Input: part model. Units: mm. Frame: model coordinates. Face numbers are marked on the shaded views. A direction names the side the tool comes from. Round coordinates to 2 decimals unless told otherwise and drop trailing zeros. Loops run counter-clockwise (first coordinate to the right, second up) from the corner with the lowest first, then second, coordinate; pieces in that order, holes last.
(1) Cut plane D-D, the plane z = -2.3. Output: boundary loops of the cut face in (x, y), and give its area (3 significant figures).
(2) Line query: line 1 (Y direction, x = -8, z = 1.85); line 2 (Y direction, x = 6.5, z = 0.9); line 3 (Z direction, x = 4, y = 4.5). Output: solid intervals per line, ascending.
(3) Cut plane A-A, the plane y = 0. Output: boundary loops of the cut face in (x, z), and give its area (3 significant figures).
(4) Access query for the marked faces 4, 5 and 6. Directions: +Z, -Z, +X, -X, +Y, -Y. A direction counts if a zero-diameter tool reaches every point of the face in a straight line with its end or side. Return the directions, or none.
(5) First-contact query: pin 1 Ø6 at (x, y) = (-5.5, 4) entering from +Z; pin 2 Ø4.5 at (x, y) = (-0.5, -1) entering from -Z; pin 3 Ø3 at (x, y) = (0, -7.25) entering from +Z; pin 4 Ø3 at (x, z) = (3.5, 0.5) entering from +Y. Flat tips, straight axial feed; report the tip coordinate or a pass-through.
(6) Draft query along X for the marked faces 1, 2 and 3. Return one class per face: released by +X, released by -X, zero draft, split by the parting line, or undercut.
(7) Cut plane C-C, the plane z = 1.1. Give the number of separate pieces and of enclosed holes in the cut face, and give its area (3 significant figures).
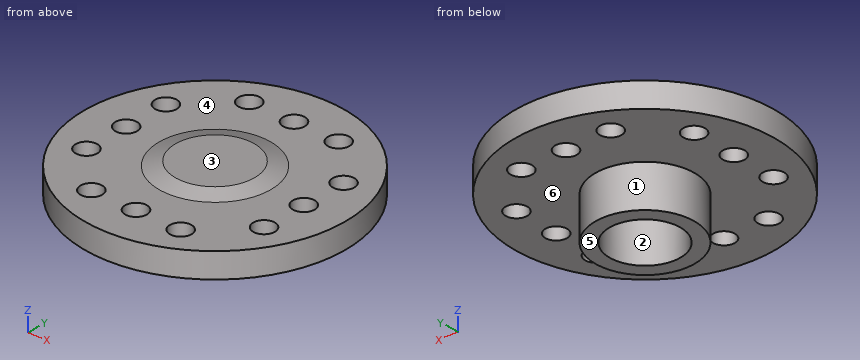
from build123d import *

# Parameters (mm, degrees)
ESQUISSE1_R             = 10.5
ESQUISSE1_R_2           = 0.875
BOSS_EXTRU_1_DEPTH      = 2
ESQUISSE2_R             = 4.5
BOSS_EXTRU_2_DEPTH      = 0.35
BOSS_EXTRU_2_TAPER      = 75
ESQUISSE3_R             = 4
BOSS_EXTRU_3_DEPTH      = 3.4
ESQUISSE4_R             = 2.85
ENL_V_MAT_EXTRU_1_DEPTH = 3.8


with BuildPart() as part:
    # Esquisse1 → Boss.-Extru.1 (new body)
    with BuildSketch(Plane.XY):
        Circle(ESQUISSE1_R)
        with Locations((7.2545, 3.65)):
            Circle(ESQUISSE1_R_2, mode=Mode.SUBTRACT)
        with Locations((7.2545, 0)):
            Circle(ESQUISSE1_R_2, mode=Mode.SUBTRACT)
        with Locations(Location((7.2545, -3.65, 0), (0, 0, 180))):
            Circle(ESQUISSE1_R_2, mode=Mode.SUBTRACT)
        with Locations((3.65, -7.2545)):
            Circle(ESQUISSE1_R_2, mode=Mode.SUBTRACT)
        with Locations((0, -7.2545)):
            Circle(ESQUISSE1_R_2, mode=Mode.SUBTRACT)
        with Locations(Location((-3.65, -7.2545, 0), (0, 0, 180))):
            Circle(ESQUISSE1_R_2, mode=Mode.SUBTRACT)
        with Locations((-7.2545, -3.65)):
            Circle(ESQUISSE1_R_2, mode=Mode.SUBTRACT)
        with Locations((-7.2545, 0)):
            Circle(ESQUISSE1_R_2, mode=Mode.SUBTRACT)
        with Locations(Location((-7.2545, 3.65, 0), (0, 0, 180))):
            Circle(ESQUISSE1_R_2, mode=Mode.SUBTRACT)
        with Locations((-3.65, 7.2545)):
            Circle(ESQUISSE1_R_2, mode=Mode.SUBTRACT)
        with Locations((0, 7.2545)):
            Circle(ESQUISSE1_R_2, mode=Mode.SUBTRACT)
        with Locations(Location((3.65, 7.2545, 0), (0, 0, 180))):
            Circle(ESQUISSE1_R_2, mode=Mode.SUBTRACT)
    extrude(amount=BOSS_EXTRU_1_DEPTH)

    # Esquisse2 → Boss.-Extru.2 (add)
    with BuildSketch(Plane.XY.offset(2)):
        Circle(ESQUISSE2_R)
    extrude(amount=BOSS_EXTRU_2_DEPTH, taper=BOSS_EXTRU_2_TAPER)

    # Esquisse3 → Boss.-Extru.3 (add)
    with BuildSketch(Plane(origin=(0, 0, 0), x_dir=(-1, 0, 0), z_dir=(0, 0, -1))):
        with Locations(Location((0, 0, 0), (0, 0, 180))):
            Circle(ESQUISSE3_R)
    extrude(amount=BOSS_EXTRU_3_DEPTH)

    # Esquisse4 → Enlèv. mat.-Extru.1 (cut)
    with BuildSketch(Plane(origin=(0, 0, -3.4), x_dir=(-1, 0, 0), z_dir=(0, 0, -1))):
        Circle(ESQUISSE4_R)
    extrude(amount=-ENL_V_MAT_EXTRU_1_DEPTH, mode=Mode.SUBTRACT)


solid = part.part
Reported:
1. outline: circle Ø8 at (0, 0); hole circle Ø5.7 at (0, 0)
1. area: 24.7 mm2
2. line 1: y = -6.8 to -4.11, -3.19 to -0.46, 0.46 to 3.19, 4.11 to 6.8
2. line 2: y = -8.25 to -4.09, -3.21 to -0.44, 0.44 to 3.21, 4.09 to 8.25
2. line 3: z = 0 to 2
3. outline: (-10.5, 0) - (-8.13, 0) - (-8.13, 2) - (-10.5, 2) - close; (-6.38, 0) - (-4, 0) - (-4, -3.4) - (-2.85, -3.4) - (-2.85, 0.4) - (2.85, 0.4) - (2.85, -3.4) - (4, -3.4) - (4, 0) - (6.38, 0) - (6.38, 2) - (4.5, 2) - (3.19, 2.35) - (-3.19, 2.35) - (-4.5, 2) - (-6.38, 2) - close; (8.13, 0) - (10.5, 0) - (10.5, 2) - (8.13, 2) - close
3. area: 43.2 mm2
4. face 4: +Z
4. face 5: -Z, +X, -X, +Y, -Y
4. face 6: -Z
5. pin 1: stops at z = 2.19
5. pin 2: stops at z = -3.4
5. pin 3: stops at z = 2
5. pin 4: stops at y = 10.31
6. face 1: split by the parting line
6. face 2: undercut
6. face 3: zero draft
7. separate pieces: 1
7. enclosed holes: 12
7. area: 317 mm2
